from build123d import *


with BuildPart() as part:
    # Sketch2 → Revolve2 (revolve)
    with BuildSketch(Plane.XY):
        with BuildLine():
            Line((20, 120), (20, 13.692287852))
            ThreePointArc((20, 13.692287852), (12.835765664, 2.704008302), (0, 0))
            Line((0, 0), (0, 0.929650957))
            Line((0, 0.929650957), (0.184018204, 0.982922835))
            ThreePointArc((0.184018204, 0.982922835), (12.233100998, 3.503391888), (19, 13.786496394))
            Line((19, 13.786496394), (19, 121))
            Line((19, 121), (27.059808742, 121))
            Line((27.059808742, 121), (27.059808742, 120))
            Line((27.059808742, 120), (20, 120))
        make_face()
    revolve(axis=Axis((0, 0, 0), (0, 1, 0)))


solid = part.part
For this review, take the finished solid that the model builds, in its own axes (mm). A direction names the side the tool comes from. Give positions to 0.01 mm unless a question says otherwise; leave off trailing zeros. Loops run counter-clockwise (first coordinate to the right, second up) from the corner with the lowest first, then second, coordinate; pieces in that order, holes last. Notation, with made-up numbers: M 30.25,-29 L 57.25,-29 A30 cw 57.25,-7 Z; hole C -28,43 d9. An arc over 180 degrees is marked long. Answer as a JSON object with one key per item and string values. Group by question number.
Q1. Add section C-C on x = -23. Give the boundary of the cut face in (y, z), and give its area (3 significant figures).
Q2. For probe 1 along Z at (x, y) = (0, 81.5); probe 2 along X at (y, z) = (65, 11), list the stretches that pass through material, from the lowest coordinate up. Write a range as [from, to].
Q3. Add section A-A on y = 106.5. Give the boundary of the cut face in (x, z).
Q4. Mouldability with a two-part tool opening along Z and no side actions: class faces 3 (the cylindrical face through (8.767, 68.144, 16.856)), 4 (the cylindrical face through (-4.336, 66.102, 19.524)), 5 (the flat face through (-5.6, 121, -18.4)) as +Z half, -Z half, draft (parallel to the pull), parting line (faces both ways), or undercut.
Q5. Insertion check: P1, Ø1.5, axis at x = -19, y = 63.5, coming from the -Z side; P2, Ø12, axis at y = 19.5, z = -9, coming from the -X side; P3, Ø1, axis at x = -18, y = 16, coming from the +Z side. Each pin has a flat end and moves straight along its axis. Give the tip position at first contact, or say it passes through.
Q6. Add section B-B on z = 23. Give the boundary of the cut face in (x, y), and give its area (3 significant figures).
Q7. Tool access review of faces 1 (the flat face through (-10, 120, 18)), 2 (the cylindrical face through (-3.52, 120.49, -26.83)): name each direction out of +Z, -Z, +X, -X, +Y, -Y from which nothing blocks a thin tool from reaching the whole face with its end or side.
Checked values:
{
 "1": {"outline": "M 120,-14.26 L 121,-14.26 L 121,14.26 L 120,14.26 Z", "area": "28.5 mm²"},
 "2": {"probe 1": "[-20, -19], [19, 20]", "probe 2": "[-16.7, -15.49], [15.49, 16.7]"},
 "3": {"outline": "C 0,0 d40; hole C 0,0 d38"},
 "4": {"face 3": "undercut", "face 4": "parting line", "face 5": "draft"},
 "5": {"P1": "z = -8.18", "P2": "x = -19.77", "P3": "z = 9.68"},
 "6": {"outline": "M -14.26,120 L 14.26,120 L 14.26,121 L -14.26,121 Z", "area": "28.5 mm²"},
 "7": {"face 1": "-Y", "face 2": "+Y, -Y"}
}
